Geometry: final body of the model. Coordinates: model frame, mm. Coordinates: 2 decimals unless noted, no trailing zeros. Write each loop counter-clockwise with the first axis right and the second up, starting at its lowest first coordinate (ties: lowest second). Pieces come first, ordered by that corner, then holes. Notation, with made-up numbers: (76.25, 49.5) -> (105.25, 49.5) arc R21 cw to (105.25, 77.5) -> close; hole circle Ø1 at (63.5, 46.5). An arc over 180 degrees is marked (long way). One line per item, written item: value.
```python
from build123d import *

# Parameters (mm, degrees)
MODEL_W                 = 3
MODEL_H                 = 3
SALIENTE_EXTRUIR1_DEPTH = 3


with BuildPart() as part:
    # Model → Saliente-Extruir1 (new body)
    with BuildSketch(Plane.XY):
        with BuildLine():
            Line((13.912774389, 239.757149551), (103.912774389, 239.757149551))
            ThreePointArc((103.912774389, 239.757149551), (107.094754904, 241.075169036), (108.412774389, 244.257149551))
            Line((108.412774389, 244.257149551), (108.412774389, 289.257149551))
            ThreePointArc((108.412774389, 289.257149551), (107.094754904, 292.439130067), (103.912774389, 293.757149551))
            Line((103.912774389, 293.757149551), (38.276735419, 293.757149551))
            ThreePointArc((38.276735419, 293.757149551), (36.554659974, 293.414607448), (35.094754904, 292.439130067))
            Line((35.094754904, 292.439130067), (10.730793873, 268.075169036))
            ThreePointArc((10.730793873, 268.075169036), (9.755316492, 266.615263966), (9.412774389, 264.893188521))
            Line((9.412774389, 264.893188521), (9.412774389, 244.257149551))
            ThreePointArc((9.412774389, 244.257149551), (10.730793873, 241.075169036), (13.912774389, 239.757149551))
        make_face()
        with Locations((13.912774389, 253.257149551)):
            Rectangle(MODEL_W, MODEL_H, mode=Mode.SUBTRACT)
        with Locations((103.912774389, 244.257149551)):
            Rectangle(MODEL_W, MODEL_H, mode=Mode.SUBTRACT)
        with Locations((103.912774389, 289.257149551)):
            Rectangle(MODEL_W, MODEL_H, mode=Mode.SUBTRACT)
        with Locations((58.912774389, 289.257149551)):
            Rectangle(MODEL_W, MODEL_H, mode=Mode.SUBTRACT)
        with Locations((103.912774389, 253.257149551)):
            Rectangle(MODEL_W, MODEL_H, mode=Mode.SUBTRACT)
        with Locations((103.912774389, 280.257149551)):
            Rectangle(MODEL_W, MODEL_H, mode=Mode.SUBTRACT)
        with Locations((67.912774389, 289.257149551)):
            Rectangle(MODEL_W, MODEL_H, mode=Mode.SUBTRACT)
        with Locations((49.912774389, 289.257149551)):
            Rectangle(MODEL_W, MODEL_H, mode=Mode.SUBTRACT)
        with Locations((103.912774389, 271.257149551)):
            Rectangle(MODEL_W, MODEL_H, mode=Mode.SUBTRACT)
        with Locations((103.912774389, 262.257149551)):
            Rectangle(MODEL_W, MODEL_H, mode=Mode.SUBTRACT)
        with Locations((58.912774389, 244.257149551)):
            Rectangle(MODEL_W, MODEL_H, mode=Mode.SUBTRACT)
        with Locations((67.912774389, 244.257149551)):
            Rectangle(MODEL_W, MODEL_H, mode=Mode.SUBTRACT)
        with Locations((49.912774389, 244.257149551)):
            Rectangle(MODEL_W, MODEL_H, mode=Mode.SUBTRACT)
        with Locations((13.912774389, 244.257149551)):
            Rectangle(MODEL_W, MODEL_H, mode=Mode.SUBTRACT)
        with Locations((13.912774389, 262.257149551)):
            Rectangle(MODEL_W, MODEL_H, mode=Mode.SUBTRACT)
    extrude(amount=SALIENTE_EXTRUIR1_DEPTH)


solid = part.part
```
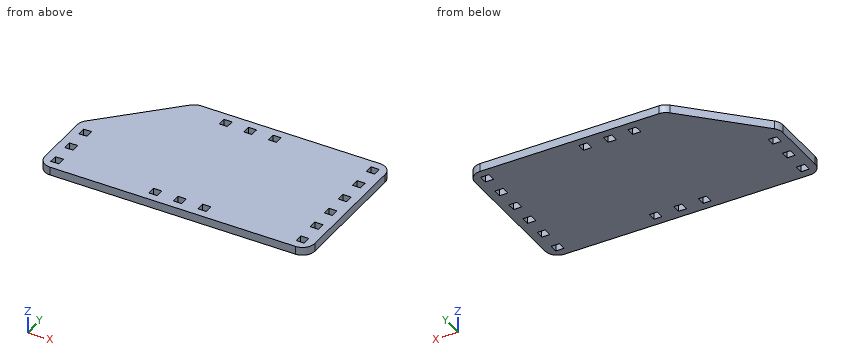
(1) First-contact query: pin 1 (1.5 mm diameter, centred on y = 290, z = 1, fed in from -X). Flat tip, straight axial feed; report the tip coordinate or a pass-through.
Responses:
pin 1: stops at x = 31.91
(2) Section A-A (z = 1.95). State how many separate pieces and enclosed holes the cut face has, then the cut area to 3 significant figures.
Responses:
separate pieces: 1
enclosed holes: 15
area: 4,830 mm2
(3) Line query: line 1 (Y direction, x = 49.5, z = 1.75); line 2 (Y direction, x = 38, z = 0.4); line 3 (X direction, y = 286, z = 1.2). Output: solid intervals per line, ascending. Write a range as [from, to].
Responses:
line 1: y = [239.76, 242.76], [245.76, 287.76], [290.76, 293.76]
line 2: y = [239.76, 293.75]
line 3: x = [28.66, 108.41]
(4) Section B-B (x = 24.5). Return the cut outline in (y, z), then the cut area to 3 significant figures.
Responses:
outline: (239.76, 0) -> (281.84, 0) -> (281.84, 3) -> (239.76, 3) -> close
area: 126 mm2
